from build123d import *

# Parameters (mm, degrees)
SKETCH1_W            = 19.05
SKETCH1_H            = 31.75
EXTRUDE1_DEPTH       = 6.35
SKETCH3_W            = 6.35
SKETCH3_H            = 31.75
EXTRUDE2_DEPTH       = 85.9886012
SKETCH4_W            = 6.35
SKETCH4_H            = 29.718
EXTRUDE3_DEPTH       = 21.59
SKETCH5_W            = 6.35
SKETCH5_H            = 29.718
EXTRUDE4_DEPTH       = 39.399
M4_CLEARANCE_HOLE1_D = 4.5
M4_CLEARANCE_HOLE2_D = 4.5


with BuildPart() as part:
    # Sketch1 → Extrude1 (new body)
    with BuildSketch(Plane(origin=(0, 0, 0), x_dir=(1, 0, 0), z_dir=(0, 1, 0))):
        Rectangle(SKETCH1_W, SKETCH1_H)
    extrude(amount=EXTRUDE1_DEPTH)

    # Sketch3 → Extrude2 (add)
    with BuildSketch(Plane(origin=(0, 6.35, 0), x_dir=(1, 0, 0), z_dir=(0, 1, 0))):
        with Locations((-6.35, 0)):
            Rectangle(SKETCH3_W, SKETCH3_H)
    extrude(amount=EXTRUDE2_DEPTH)

    # Sketch4 → Extrude3 (add)
    with BuildSketch(Plane(origin=(0, 0, -15.875), x_dir=(-1, 0, 0), z_dir=(0, 0, -1))):
        with Locations((6.35, 77.4796012)):
            Rectangle(SKETCH4_W, SKETCH4_H)
    extrude(amount=EXTRUDE3_DEPTH)

    # Sketch5 → Extrude4 (add)
    with BuildSketch(Plane.ZY.offset(9.525)):
        with Locations((-34.29, 77.4796012)):
            Rectangle(SKETCH5_W, SKETCH5_H)
    extrude(amount=EXTRUDE4_DEPTH)

    # M4 Clearance Hole1 (through all)
    with Locations(Plane(origin=(30.89, -14.85899888, -37.465), x_dir=(-1, 0, 0), z_dir=(0, 0, -1))):
        with Locations((71.305, 85.98860008), (58.605, 85.98860008), (58.605, 98.68860008), (71.305, 98.68860008)):
            Hole(M4_CLEARANCE_HOLE1_D / 2)

    # M4 Clearance Hole2 (through all)
    with Locations(Plane(origin=(0, 6.35, 0), x_dir=(-1, 0, 0), z_dir=(0, 1, 0))):
        with Locations((-3.175, 6.313141271), (-3.175, -6.956578863)):
            Hole(M4_CLEARANCE_HOLE2_D / 2)


solid = part.part
Input: part model. Units: mm. Frame: model coordinates. A direction names the side the tool comes from. Give positions to 0.01 mm unless a question says otherwise; leave off trailing zeros. Loops run counter-clockwise (first coordinate to the right, second up) from the corner with the lowest first, then second, coordinate; pieces in that order, holes last. Notation, with made-up numbers: (-37, -11.75) - (20, -11.75) arc R23 cw to (20, 12.25) - close; hole circle Ø3 at (4.25, 29). An arc over 180 degrees is marked (long way). Use CSV: the item, a comma, the result in double quotes. Start each with the question number.
Item 1: Contact query for flat-ended pins moving along their axis: P1, Ø12, axis at x = -36, z = -30.5, coming from the -Y side; P2, Ø6, axis at x = -27.71, y = 83.83, coming from the -Z side (3 decimals); P3, Ø9.5, axis at x = 0, y = 33.5, coming from the -Z side (3 decimals); P4, Ø6, axis at x = 3.18, z = 6.31, coming from the +Y side. Output: stop coordinate, or through.
Item 2: Line query: line 1 (Y direction, x = -39.5, z = -32); line 2 (X direction, y = 52, z = -3) (3 decimals); line 3 (Z direction, x = -5.5, y = 36.5) (3 decimals). Output: solid intervals per line, ascending.
Item 3: Section A-A on x = 4. Return loops of the section in (y, z) (3 decimals), then the cut area to 3 significant figures.
Item 4: Section D-D on x = -23. Return loops of the section in (y, z) (3 decimals).
Item 5: Section B-B on y = 67. Return loops of the section in (x, z) (3 decimals).
Item 6: Mould query, pull axis X, two halves, no side actions, for faces 1 (the cylindrical face through (-40.903, 81.633, -34.246)), 2 (the flat face through (-9.525, 46, -2)), 3 (the cylindrical face through (-28.203, 81.633, -34.246)), 4 (the flat face through (-4, 35, 15.875)). Classes: pulls with the +X half, pulls with the -X half, needs draft (parallel to the pull), parting line crosses it, or undercut.
Item 7: Section C-C on z = 3. Return loops of the section in (x, y) (3 decimals).
Item 8: Reachability of faces 5 (the flat face through (-21, 62.621, -32)), 6 (the flat face through (3, 6.35, 0)), 7 (the flat face through (-29, 77, -31.115)), 8 (the cylindrical face through (4.213, 3.131, 4.317)) from +Z, -Z, +X, -X, +Y, -Y: full face, straight path, thin tool, end or side. Return the list, or none.
Ans:
1,P1,"stops at y = 62.62"
1,P2,"stops at z = -37.465"
1,P3,"stops at z = -15.875"
1,P4,"stops at y = 6.35"
2,line 1,"y = 62.62 to 69.07, 73.19 to 81.77, 85.89 to 92.34"
2,line 2,"x = -9.525 to -3.175"
2,line 3,"z = -15.875 to 15.875"
3,outline,"(0, -15.875) - (6.35, -15.875) - (6.35, -9.05) - (0, -9.05) - close; (0, -4.863) - (6.35, -4.863) - (6.35, 4.22) - (0, 4.22) - close; (0, 8.406) - (6.35, 8.406) - (6.35, 15.875) - (0, 15.875) - close"
3,area,"148 mm2"
4,outline,"(62.621, -37.465) - (92.339, -37.465) - (92.339, -31.115) - (62.621, -31.115) - close"
5,outline,"(-48.924, -37.465) - (-3.175, -37.465) - (-3.175, 15.875) - (-9.525, 15.875) - (-9.525, -31.115) - (-48.924, -31.115) - close"
6,face 1,"undercut"
6,face 2,"pulls with the -X half"
6,face 3,"undercut"
6,face 4,"needs draft"
7,outline,"(-9.525, 0) - (9.525, 0) - (9.525, 6.35) - (-3.175, 6.35) - (-3.175, 92.339) - (-9.525, 92.339) - close"
8,face 5,"-Z, +X, -X, -Y"
8,face 6,"+Z, -Z, +X, +Y"
8,face 7,"+Z, -X, +Y, -Y"
8,face 8,"+Y, -Y"
